Autodesk Inventor part; units mm, degrees
ref_plane "YZ Plane" through (0, 0, 0) normal (1, 0, 0) x (0, 1, 0)
ref_plane "XZ Plane" through (0, 0, 0) normal (0, 1, 0) x (-1, 0, 0)
ref_plane "XY Plane" through (0, 0, 0) normal (0, 0, 1) x (1, 0, 0)
sketch "Sketch1" plane through (0, 0, 0) normal (0, 1, 0) x (-1, 0, 0)
  arc A0 (3.3166, 5) -> (-3.3166, -5) centre (0, 0) ccw
  line L0 (3.3166, 5) -> (-3.3166, 5) construction
  line L1 (3.3166, -5) -> (-3.3166, -5) construction
  arc A1 (3.3166, 5) -> (-3.3166, 5) centre (0, 0) ccw construction
  arc A2 (3.3166, -5) -> (3.3166, 5) centre (0, 0) ccw
  arc A3 (-3.3166, -5) -> (3.3166, -5) centre (0, 0) ccw
  line L2 (0, 0) -> (18.76, 0) construction
  point P0 (5.7735, 0)
  dimension "d17" = 10
  dimension "d18" = 12
extrude "Extrusion1" add sketch "Sketch1" along normal blind 16
sketch "Sketch2" plane through (0, 0, 0) normal (0, 1, 0) x (-1, 0, 0)
  circle A0 centre (0, 0) radius 4
  dimension "d3" = 8
extrude "Extrusion2" add sketch "Sketch2" against normal blind 36
thread "Thread1"
sketch "Sketch4" plane through (0, 16, 0) normal (0, 1, 0) x (1, 0, 0)
  circle A0 centre (0, 0) radius 6 construction
  line L0 (-3.3166, -5) -> (3.3166, -5)
  line L1 (3.3166, 5) -> (-3.3166, 5)
  arc A1 (-3.3166, -5) -> (3.3166, -5) centre (0, 0) ccw
  arc A2 (3.3166, 5) -> (-3.3166, 5) centre (0, 0) ccw
  dimension "d20" = 10
extrude "Extrusion3" cut sketch "Sketch4" against normal blind 13
sketch "Sketch3" plane through (0, 16, 0) normal (0, 1, 0) x (1, 0, 0)
  point P0 (0, 0)
  point P1 (0, 0)
hole "Hole1" at (0, 16, 0) direction (0, -1, 0) diameter 6 depth 12
thread "Thread2"
properties part number "BallTransferUnit" material "Stainless Steel"
CAD build for the part. Positions are in the model's coordinates, mm. A direction names the side the tool comes from. Round coordinates to 2 decimals unless told otherwise and drop trailing zeros. Order: outer loops, then holes, each group sorted by start corner. A loop starts at its lowest first (then second) coordinate and runs counter-clockwise, first axis right, second up. Notation, with made-up numbers: (74.25, 13.5) -> (100.25, 13.5) arc R16 cw to (100.25, 40.5) -> close; hole circle Ø6 at (61.25, 13). An arc over 180 degrees is marked (long way). One line per question, with ' | ' between items.
Q1. Two-plate mould, pull along X, no slides. Class faces 5 (the cylindrical face through (0, 10, -3)), 6 (the flat face through (0, 4, 0)), 7 (the cylindrical face through (0.867, -17.748, -3.905)), 8 (the flat face through (0, 3, -5.4)): released by +X, released by -X, zero draft, split by the parting line, or undercut.
Completed:
face 5: undercut | face 6: undercut | face 7: split by the parting line | face 8: zero draft
Q2. Drop flat-ended pins along their axis: pin 1 (1.5 mm diameter, centred on y = -27.5, z = 1.5, fed in from +X); pin 2 (3.5 mm diameter, centred on x = 0, y = 6.5, fed in from -Z); pin 3 (5 mm diameter, centred on y = -16, z = -0.5, fed in from +X). Give the stop position or say it passes through.
Completed:
pin 1: stops at x = 3.93 | pin 2: stops at z = -5 | pin 3: stops at x = 4
Q3. Slice it at C-C (z = 0). Write the cut outline in (x, y).
Completed:
outline: (-6, 0) -> (-4, 0) -> (-4, -36) -> (4, -36) -> (4, 0) -> (6, 0) -> (6, 16) -> (3, 16) -> (3, 4) -> (-3, 4) -> (-3, 16) -> (-6, 16) -> close
Q4. Slice it at B-B (x = 0). Write the cut outline in (y, z), then the cut area to 3 significant figures.
Completed:
outline: (-36, -4) -> (0, -4) -> (0, -6) -> (3, -6) -> (3, -5) -> (16, -5) -> (16, -3) -> (4, -3) -> (4, 3) -> (16, 3) -> (16, 5) -> (3, 5) -> (3, 6) -> (0, 6) -> (0, 4) -> (-36, 4) -> close | area: 382 mm^2
Q5. Slice it at D-D (z = -2). Write the cut outline in (x, y), then the cut area to 3 significant figures.
Completed:
outline: (-5.66, 0) -> (-3.46, 0) -> (-3.46, -36) -> (3.46, -36) -> (3.46, 0) -> (5.66, 0) -> (5.66, 16) -> (2.24, 16) -> (2.24, 4) -> (-2.24, 4) -> (-2.24, 16) -> (-5.66, 16) -> close | area: 377 mm^2
Q6. Slice it at A-A (y = 5.5). Write the cut outline in (x, z), then the cut area to 3 significant figures.
Completed:
outline: (-3.32, -5) -> (3.32, -5) arc R6 ccw to (3.32, 5) -> (-3.32, 5) arc R6 ccw to start; hole circle Ø6 at (0, 0) | area: 75.8 mm^2
Q7. Which spindle directions (+Z, -Z, +X, -X, +Y, -Y) get a long thin tool onto all of the face, cutting with end or side? Do faces 1 (the flat face through (0, 10, -5)), 2 (the flat face through (1.42, 0, -3.92)), 3 (the flat face through (0, -36, 0)), 4 (the flat face through (0, 3, 5.4)). Say none if no direction does.
Completed:
face 1: -Z, +X, -X, +Y | face 2: -Y | face 3: +Z, -Z, +X, -X, -Y | face 4: +Z, +X, -X, +Y
Q8. Probe probe 1 along Z at (x, y) = (0, 13.75); probe 2 along X at (y, z) = (9.75, 0); probe 3 along Y at (x, z) = (2.25, 3.75). List the from-to ranges inside material, lowest first.
Completed:
probe 1: z = -5 to -3, 3 to 5 | probe 2: x = -6 to -3, 3 to 6 | probe 3: y = 0 to 16
